```python
from build123d import *

# Parameters (mm, degrees)
SKETCH1_W               = 170
SKETCH1_H               = 40
BOSS_EXTRUDE1_DEPTH     = 3
SKETCH3_W               = 3
SKETCH3_H               = 6
BOSS_EXTRUDE2_DEPTH     = 3
LPATTERN1_COUNT         = 3
LPATTERN1_PITCH         = 12
LPATTERN1_COL_COUNT     = 2
LPATTERN1_COL_PITCH     = 12
SKETCH4_W               = 3
SKETCH4_H               = 6
BOSS_EXTRUDE3_DEPTH     = 3
LPATTERN2_COUNT         = 8
LPATTERN2_PITCH         = 12
LPATTERN2_COL_COUNT     = 8
LPATTERN2_COL_PITCH     = 12
MIRROR1_COPY_1_SKETCH_W = 3
MIRROR1_COPY_1_SKETCH_H = 6
MIRROR1_COPY_1_DEPTH    = 3
MIRROR1_COPY_2_SKETCH_W = 3
MIRROR1_COPY_2_SKETCH_H = 6
MIRROR1_COPY_2_DEPTH    = 3
MIRROR1_COPY_3_SKETCH_W = 3
MIRROR1_COPY_3_SKETCH_H = 6
MIRROR1_COPY_3_DEPTH    = 3
SKETCH6_R               = 1
SKETCH6_W               = 24
SKETCH6_H               = 13
CUT_EXTRUDE2_DEPTH      = 4
SKETCH7_W               = 3
SKETCH7_H               = 3
CUT_EXTRUDE4_DEPTH      = 4
SKETCH8_W               = 3
SKETCH8_H               = 1
CUT_EXTRUDE5_DEPTH      = 3


with BuildPart() as part:
    # Sketch1 → Boss-Extrude1 (new body)
    with BuildSketch(Plane(origin=(0, 0, 0), x_dir=(0, 0, -1), z_dir=(1, 0, 0))):
        Rectangle(SKETCH1_W, SKETCH1_H)
    extrude(amount=BOSS_EXTRUDE1_DEPTH)

    # Sketch3 → Boss-Extrude2 (add)
    with BuildSketch(Plane(origin=(0, 0, -85), x_dir=(-1, 0, 0), z_dir=(0, 0, -1))):
        with Locations((-1.5, 6)):
            Rectangle(SKETCH3_W, SKETCH3_H)
    boss_extrude2 = extrude(amount=BOSS_EXTRUDE2_DEPTH)

    # LPattern1: Boss-Extrude2 ×3
    with Locations(*[(0, -i * LPATTERN1_PITCH, 0) for i in range(1, LPATTERN1_COUNT)]):
        add(boss_extrude2)

    # LPattern1 col: Boss-Extrude2 ×2
    with Locations(*[(0, i * LPATTERN1_COL_PITCH, 0) for i in range(1, LPATTERN1_COL_COUNT)]):
        add(boss_extrude2)

    # Sketch4 → Boss-Extrude3 (add)
    with BuildSketch(Plane(origin=(0, 20, 0), x_dir=(1, 0, 0), z_dir=(0, 1, 0))):
        with Locations((1.5, 0)):
            Rectangle(SKETCH4_W, SKETCH4_H)
    boss_extrude3 = extrude(amount=BOSS_EXTRUDE3_DEPTH)

    # LPattern2: Boss-Extrude3 ×8
    with Locations(*[(0, 0, -i * LPATTERN2_PITCH) for i in range(1, LPATTERN2_COUNT)]):
        add(boss_extrude3)

    # LPattern2 col: Boss-Extrude3 ×8
    with Locations(*[(0, 0, i * LPATTERN2_COL_PITCH) for i in range(1, LPATTERN2_COL_COUNT)]):
        add(boss_extrude3)

    # Mirror1: Boss-Extrude2 across plane
    add(boss_extrude2.mirror(Plane.XY))

    # Mirror1 copy 1 sketch → Mirror1 copy 1 (add)
    with BuildSketch(Plane(origin=(0, -12, 85), x_dir=(-1, 0, 0), z_dir=(0, 0, 1))):
        with Locations((-1.5, -6)):
            Rectangle(MIRROR1_COPY_1_SKETCH_W, MIRROR1_COPY_1_SKETCH_H)
    extrude(amount=MIRROR1_COPY_1_DEPTH)

    # Mirror1 copy 2 sketch → Mirror1 copy 2 (add)
    with BuildSketch(Plane(origin=(0, -24, 85), x_dir=(-1, 0, 0), z_dir=(0, 0, 1))):
        with Locations((-1.5, -6)):
            Rectangle(MIRROR1_COPY_2_SKETCH_W, MIRROR1_COPY_2_SKETCH_H)
    extrude(amount=MIRROR1_COPY_2_DEPTH)

    # Mirror1 copy 3 sketch → Mirror1 copy 3 (add)
    with BuildSketch(Plane(origin=(0, 12, 85), x_dir=(-1, 0, 0), z_dir=(0, 0, 1))):
        with Locations((-1.5, -6)):
            Rectangle(MIRROR1_COPY_3_SKETCH_W, MIRROR1_COPY_3_SKETCH_H)
    extrude(amount=MIRROR1_COPY_3_DEPTH)

    # Sketch6 → Cut-Extrude2 (cut, through all)
    with BuildSketch(Plane(origin=(3, 0, 0), x_dir=(0, 0, -1), z_dir=(1, 0, 0))):
        with Locations((28.1, -5.368175576)):
            Circle(SKETCH6_R)
        with Locations((55.9, -5.368175576)):
            Circle(SKETCH6_R)
        with Locations((28.1, 9.494198583)):
            Circle(SKETCH6_R)
        with Locations((55.9, 9.494198583)):
            Circle(SKETCH6_R)
        with Locations((42, -5.368175576)):
            Rectangle(SKETCH6_W, SKETCH6_H)
        with Locations((42, 9.494198583)):
            Rectangle(SKETCH6_W, SKETCH6_H)
    extrude(amount=-CUT_EXTRUDE2_DEPTH, mode=Mode.SUBTRACT)

    # Sketch7 → Cut-Extrude4 (cut, through all)
    with BuildSketch(Plane(origin=(3, 0, 0), x_dir=(0, 0, -1), z_dir=(1, 0, 0))):
        with Locations((86.5, 21.5)):
            Rectangle(SKETCH7_W, SKETCH7_H)
    cut_extrude4 = extrude(amount=-CUT_EXTRUDE4_DEPTH, mode=Mode.SUBTRACT)

    # Mirror2: Cut-Extrude4 across plane
    add(cut_extrude4.mirror(Plane.XY), mode=Mode.SUBTRACT)

    # Sketch8 → Cut-Extrude5 (cut)
    with BuildSketch(Plane.ZY):
        with Locations((86.5, -20.5)):
            Rectangle(SKETCH8_W, SKETCH8_H)
    cut_extrude5 = extrude(amount=-CUT_EXTRUDE5_DEPTH, mode=Mode.SUBTRACT)

    # Mirror3: Cut-Extrude5 across plane
    add(cut_extrude5.mirror(Plane.XY), mode=Mode.SUBTRACT)


solid = part.part
```
Work out the finished part from the listing and answer in its coordinate system (mm). A direction names the side the tool comes from. Round coordinates to 2 decimals unless told otherwise and drop trailing zeros. Order: outer loops, then holes, each group sorted by start corner. A loop starts at its lowest first (then second) coordinate and runs counter-clockwise, first axis right, second up.
Q1. A tool of negligible diameter and unlimited length cuts with its end or side. For faces 4 (the flat face through (1, 21, -63)), 5 (the flat face through (2, 1.132, -42)), 6 (the flat face through (2, -9, 86)), 7 (the flat face through (1, 23, 83)), 8 (the flat face through (2, 3, -86)), from which of +Z, -Z, +X, -X, +Y, -Y can it reach the whole face along a straight path? Write none if from no direction.
Solution:
face 4: +X, -X, +Y
face 5: +X, -X
face 6: +Z, +X, -X
face 7: +Z, -Z, +X, -X, +Y
face 8: -Z, +X, -X
Q2. The mould has two halves that part along Z. Classify faces 1 (the flat face through (1, 23, -48)), 2 (the flat face through (1, -12, -85)), 3 (the flat face through (2, 15.994, -42)): pulls with the +Z half, pulls with the -Z half, needs draft (parallel to the pull), parting line crosses it, or undercut.
Solution:
face 1: needs draft
face 2: pulls with the -Z half
face 3: undercut
Q3. A cutting plane is placed at B-B, the plane x = 2.2. Count the separate pieces of the cut face and the enclosed holes in it, then the cut area to 3 significant figures.
Solution:
separate pieces: 1
enclosed holes: 6
area: 6,550 mm2
Q4. A cutting plane is placed at A-A, the plane z = -52.5. Determine the outline of the cut face in (x, y), then the cut area to 3 significant figures.
Solution:
outline: (0, -20) - (3, -20) - (3, -11.87) - (0, -11.87) - close; (0, 1.13) - (3, 1.13) - (3, 2.99) - (0, 2.99) - close; (0, 15.99) - (3, 15.99) - (3, 20) - (0, 20) - close
area: 42.0 mm2
Q5. Find the intervals of material crossed by line 1 along Y through (x, z) = (0.7, -28.1); line 2 along Y through (x, z) = (1.9, -38); line 3 along Z through (x, y) = (0.65, 9.5), in increasing order.
Solution:
line 1: y = -20 to -6.37, -4.37 to 8.49, 10.49 to 20
line 2: y = -20 to -11.87, 1.13 to 2.99, 15.99 to 23
line 3: z = -85 to -56.9, -54.9 to -54, -30 to -29.1, -27.1 to 85
Q6. Given pin 1 Ø0.9 at (x, z) = (1, 43) entering from +Y; pin 2 Ø1.5 at (x, y) = (1.5, 21) entering from +Z, each flat-ended and moving along its own axis, determine where each tip first touches the part or whether it passes through.
Solution:
pin 1: stops at y = 20
pin 2: stops at z = 85
